Build history of the part. All positions in model axes, mm. A direction names the side the tool comes from. Round coordinates to 2 decimals unless told otherwise and drop trailing zeros. Write each loop counter-clockwise with the first axis right and the second up, starting at its lowest first coordinate (ties: lowest second). Pieces come first, ordered by that corner, then holes. Notation, with made-up numbers: (-30, -35.5) -> (26, -35.5) arc R28 ccw to (26, -8.5) -> close; hole circle Ø1 at (65, -22). An arc over 180 degrees is marked (long way). Answer in a Markdown table with one row per item.
```python
from build123d import *

# Parameters (mm, degrees)
BOSS_EXTRUDE1_DEPTH = 1.27
CUT_EXTRUDE1_DEPTH  = 0.635
SKETCH3_R           = 1.778
CUT_EXTRUDE2_DEPTH  = 96.027914425


with BuildPart() as part:
    # Sketch1 → Boss-Extrude1 (new body)
    with BuildSketch(Plane.XY):
        Polygon((0, 0), (12.192, 0), (12.192, -11.684), (8.509, -11.684), (8.509, -89.789), (7.0485, -94.234), (5.1435, -94.234), (3.683, -89.789), (3.683, -11.684), (0, -11.684), align=None)
    extrude(amount=BOSS_EXTRUDE1_DEPTH)

    # Sketch2 → Cut-Extrude1 (cut)
    with BuildSketch(Plane.XY.offset(1.27)):
        Polygon((5.1435, -94.234), (5.1435, -11.684), (3.683, -11.684), (3.683, -89.789), align=None)
        Polygon((8.509, -11.684), (8.509, -89.789), (7.0485, -94.234), (7.0485, -11.684), align=None)
    extrude(amount=-CUT_EXTRUDE1_DEPTH, mode=Mode.SUBTRACT)

    # Sketch3 → Cut-Extrude2 (cut, through all)
    with BuildSketch(Plane.XY.offset(1.27)):
        with Locations((6.096, -5.842)):
            Circle(SKETCH3_R)
    extrude(amount=-CUT_EXTRUDE2_DEPTH, mode=Mode.SUBTRACT)


solid = part.part
```
Q1. Saw through at C-C on x = 10. Write the cut outline in (y, z).
A:
| item | result |
|---|---|
| outline | (-11.68, 0) -> (0, 0) -> (0, 1.27) -> (-11.68, 1.27) -> close |
Q2. Saw through at A-A on y = -87. Write the cut outline in (x, z) (1 decimal), plus the area to 3 significant figures.
A:
| item | result |
|---|---|
| outline | (3.7, 0) -> (8.5, 0) -> (8.5, 0.6) -> (7, 0.6) -> (7, 1.3) -> (5.1, 1.3) -> (5.1, 0.6) -> (3.7, 0.6) -> close |
| area | 4.27 mm² |
Q3. Which spindle directions (+Z, -Z, +X, -X, +Y, -Y) get a long thin tool onto all of the face, cutting with end or side? Do faces 4 (the flat face through (7.79, -91.98, 0.31)), 5 (the flat face through (4, -52, 0.635)). Say none if no direction does.
A:
| item | result |
|---|---|
| face 4 | +Z, -Z, +X, -Y |
| face 5 | +Z, -X, -Y |
Q4. Wall check: line 1 (X direction, y = -44.5, z = 0.7); line 2 (Z direction, x = 7.75, y = -63) (3 decimals); line 3 (X direction, y = -6, z = 0.9). Give the ranges that are in metal, low to high. Write a range as [from, to].
A:
| item | result |
|---|---|
| line 1 | [5.14, 7.05] |
| line 2 | [0, 0.635] |
| line 3 | [0, 4.33], [7.87, 12.19] |
Q5. Drop a flat-ended pin along its axis: P1, Ø0.6, axis at x = 10, z = 1, coming from the -Y side. Give the stop position or say it passes through.
A:
| item | result |
|---|---|
| P1 | y = -11.68 |
Q6. Two-plate mould, pull along Y, no slides. Class faces 1 (the flat face through (4.423, -92.043, 0.313)), 2 (the flat face through (8, -52, 0.635)), 3 (the cylindrical face through (4.786, -4.64, 0.644)): released by +Y, released by -Y, zero draft, split by the parting line, or undercut.
A:
| item | result |
|---|---|
| face 1 | released by -Y |
| face 2 | zero draft |
| face 3 | undercut |
Q7. Saw through at B-B on z = 0.9. Write the cut outline in (x, y), plus the area to 3 significant figures.
A:
| item | result |
|---|---|
| outline | (0, -11.68) -> (5.14, -11.68) -> (5.14, -94.23) -> (7.05, -94.23) -> (7.05, -11.68) -> (12.19, -11.68) -> (12.19, 0) -> (0, 0) -> close; hole circle Ø3.56 at (6.1, -5.84) |
| area | 290 mm² |
